The model under review builds one solid part; all positions refer to its coordinate system, in mm. Round coordinates to 2 decimals unless told otherwise and drop trailing zeros. Order: outer loops, then holes, each group sorted by start corner. A loop starts at its lowest first (then second) coordinate and runs counter-clockwise, first axis right, second up. Notation, with made-up numbers: M -26.5,7.25 L -20.5,7.25 A26 cw -20.5,25.25 Z; hole C 8.25,4.5 d9. An arc over 180 degrees is marked long. Answer as a JSON object with one key per item and string values. Group by question number.
1. Add section B-B on z = 1.45. Give the number of separate pieces and of enclosed holes in the cut face, and give its area (3 significant figures).
2. Add section A-A on x = 117.5. State the section outline as (y, z) points (3 decimals).
3. To check wall thickness, follow probe 1 along Y at (x, z) = (89.5, 3.9); probe 2 along Y at (x, z) = (222, 2.4); probe 3 along Y at (x, z) = (42, 0.85). State the ranges of each line that lie inside material, in increasing order. Write a range as [from, to].
4. Clearance check with flat-ended pins moving along their axes: P1, Ø3, axis at x = 288.5, z = 3.5, coming from the -Y side (3 decimals); P2, Ø1.7, axis at y = 149, z = 4, coming from the -X side; P3, Ø1.7, axis at y = 143, z = 2, coming from the -X side. State where each tip first meets the part, or that it passes through.
```python
from build123d import *

# Parameters (mm, degrees)
BOSS_EXTRUDE1_DEPTH = 5.715


with BuildPart() as part:
    # Model → Boss-Extrude1 (new body)
    with BuildSketch(Plane.XY):
        Polygon((16.114776, 23.2006394), (38.974776, 23.2006394), (39.713662, 23.2006394), (41.932098, 23.590631), (44.254166, 24.4808502), (44.689776, 24.7316498), (45.123862, 24.983821), (47.05604, 26.54935), (48.622712, 28.481274), (48.87341, 28.91536), (49.124362, 29.350716), (50.690018, 31.282894), (52.621688, 32.848296), (53.057044, 33.098994), (53.491384, 33.349946), (55.813198, 34.241486), (58.031888, 34.630106), (58.772044, 34.630106), (243.457984, 34.630106), (244.196616, 34.630106), (246.415306, 34.241486), (248.737374, 33.349946), (249.172476, 33.098994), (249.606816, 32.848296), (251.53874, 31.282894), (253.105666, 29.350716), (253.356618, 28.91536), (253.607316, 28.481274), (255.17348, 26.54935), (257.10388, 24.983821), (257.54076, 24.7316498), (257.9751, 24.4808502), (260.29666, 23.590631), (262.51408, 23.2006394), (263.25576, 23.2006394), (286.11576, 23.2006394), (286.11576, 35.465004), (291.83076, 35.465004), (291.83076, 46.89475), (286.11576, 46.89475), (286.11576, 58.323988), (291.83076, 58.323988), (291.83076, 69.75475), (286.11576, 69.75475), (286.11576, 86.061296), (276.32152, 95.855028), (280.36266, 99.896676), (272.28038, 107.978956), (268.2367, 103.937054), (260.15442, 112.019334), (264.1981, 116.060982), (256.11582, 124.141738), (252.07341, 120.10136), (243.992654, 128.18364), (248.033032, 132.224272), (239.951006, 140.307822), (235.909104, 136.266174), (226.115372, 146.060922), (216.248488, 146.060922), (216.248488, 151.775668), (204.81925, 151.775668), (204.81925, 146.060922), (193.388488, 146.060922), (193.388488, 151.775668), (181.958996, 151.775668), (181.958996, 146.060922), (170.529504, 146.060922), (170.529504, 151.775668), (159.098488, 151.775668), (159.098488, 146.060922), (147.66925, 146.060922), (147.66925, 151.775668), (136.238488, 151.775668), (136.238488, 146.060922), (124.808996, 146.060922), (124.808996, 151.775668), (113.379504, 151.775668), (113.379504, 146.060922), (101.948488, 146.060922), (101.948488, 151.775668), (90.51925, 151.775668), (90.51925, 146.060922), (79.088488, 146.060922), (79.088488, 151.775668), (67.658996, 151.775668), (67.658996, 146.060922), (56.229504, 146.060922), (56.229504, 151.775668), (44.798488, 151.775668), (44.798488, 146.060922), (33.36925, 146.060922), (33.36925, 151.775668), (21.938361, 151.775668), (21.938361, 146.060922), (16.114776, 146.060922), (16.114776, 136.066022), (10.4000554, 136.066022), (10.4000554, 124.63526), (16.114776, 124.63526), (16.114776, 113.205768), (10.4000554, 113.205768), (10.4000554, 101.775006), (16.114776, 101.775006), (16.114776, 90.345768), (10.4000554, 90.345768), (10.4000554, 78.916022), (16.114776, 78.916022), (16.114776, 67.48526), (10.4000554, 67.48526), (10.4000554, 56.055768), (16.114776, 56.055768), (16.114776, 44.625006), (10.4000554, 44.625006), (10.4000554, 33.195514), (16.114776, 33.195514), align=None)
        Polygon((25.3848362, 40.346122), (19.6701156, 40.346122), (19.6701156, 46.060868), (31.099506, 46.060868), (31.099506, 40.346122), align=None, mode=Mode.SUBTRACT)
        Polygon((48.245268, 40.346122), (42.530522, 40.346122), (42.530522, 46.060868), (53.95976, 46.060868), (53.95976, 40.346122), align=None, mode=Mode.SUBTRACT)
        Polygon((71.105522, 40.346122), (65.390522, 40.346122), (65.390522, 46.060868), (76.820268, 46.060868), (76.820268, 40.346122), align=None, mode=Mode.SUBTRACT)
        Polygon((93.965522, 40.346122), (88.249506, 40.346122), (88.249506, 46.060868), (99.680522, 46.060868), (99.680522, 40.346122), align=None, mode=Mode.SUBTRACT)
        Polygon((116.824506, 40.346122), (111.10976, 40.346122), (111.10976, 46.060868), (122.540522, 46.060868), (122.540522, 40.346122), align=None, mode=Mode.SUBTRACT)
        Polygon((139.68476, 40.346122), (133.970268, 40.346122), (133.970268, 46.060868), (145.399506, 46.060868), (145.399506, 40.346122), align=None, mode=Mode.SUBTRACT)
        Polygon((162.545268, 40.346122), (156.830522, 40.346122), (156.830522, 46.060868), (168.25976, 46.060868), (168.25976, 40.346122), align=None, mode=Mode.SUBTRACT)
        Polygon((185.405522, 40.346122), (179.690522, 40.346122), (179.690522, 46.060868), (191.120268, 46.060868), (191.120268, 40.346122), align=None, mode=Mode.SUBTRACT)
        Polygon((208.265522, 40.346122), (202.549506, 40.346122), (202.549506, 46.060868), (213.980522, 46.060868), (213.980522, 40.346122), align=None, mode=Mode.SUBTRACT)
        Polygon((231.124506, 40.346122), (225.40976, 40.346122), (225.40976, 46.060868), (236.840522, 46.060868), (236.840522, 40.346122), align=None, mode=Mode.SUBTRACT)
        Polygon((253.98476, 40.346122), (248.270268, 40.346122), (248.270268, 46.060868), (259.69976, 46.060868), (259.69976, 40.346122), align=None, mode=Mode.SUBTRACT)
        Polygon((276.84476, 40.346122), (271.12976, 40.346122), (271.12976, 46.060868), (282.55976, 46.060868), (282.55976, 40.346122), align=None, mode=Mode.SUBTRACT)
    extrude(amount=BOSS_EXTRUDE1_DEPTH)


solid = part.part
```
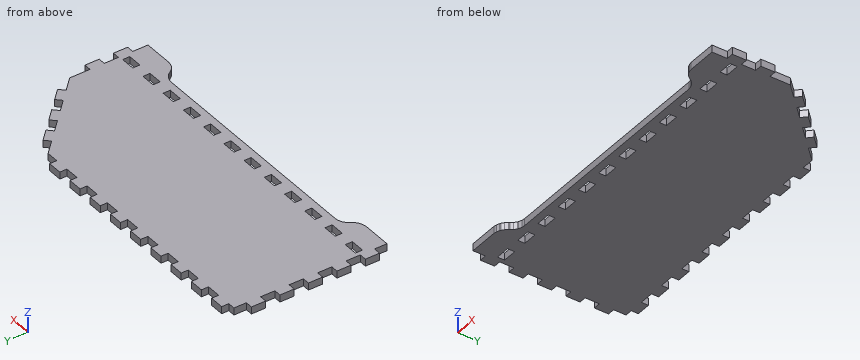
Recorded:
{
 "1": {"separate pieces": "1", "enclosed holes": "12", "area": "29,500 mm²"},
 "2": {"outline": "M 34.63,0 L 40.346,0 L 40.346,5.715 L 34.63,5.715 Z; M 46.061,0 L 151.776,0 L 151.776,5.715 L 46.061,5.715 Z"},
 "3": {"probe 1": "y = [34.63, 40.35], [46.06, 146.06]", "probe 2": "y = [34.63, 146.06]", "probe 3": "y = [23.62, 146.06]"},
 "4": {"P1": "stops at y = 35.465", "P2": "stops at x = 21.94", "P3": "stops at x = 16.11"}
}
